Could you check a few things on this drawing? It's one solid part, dimensions in mm from its lowest x, y, z. A direction names the side the tool comes from. Round coordinates to 2 decimals unless told otherwise and drop trailing zeros. Loops run counter-clockwise (first coordinate to the right, second up) from the corner with the lowest first, then second, coordinate; pieces in that order, holes last. Notation, with made-up numbers: M 77,31 L 125,31 A23 cw 125,50 Z; hole C -38,82.5 d8. An arc over 180 degrees is marked long. Answer as CSV lines item,"result".
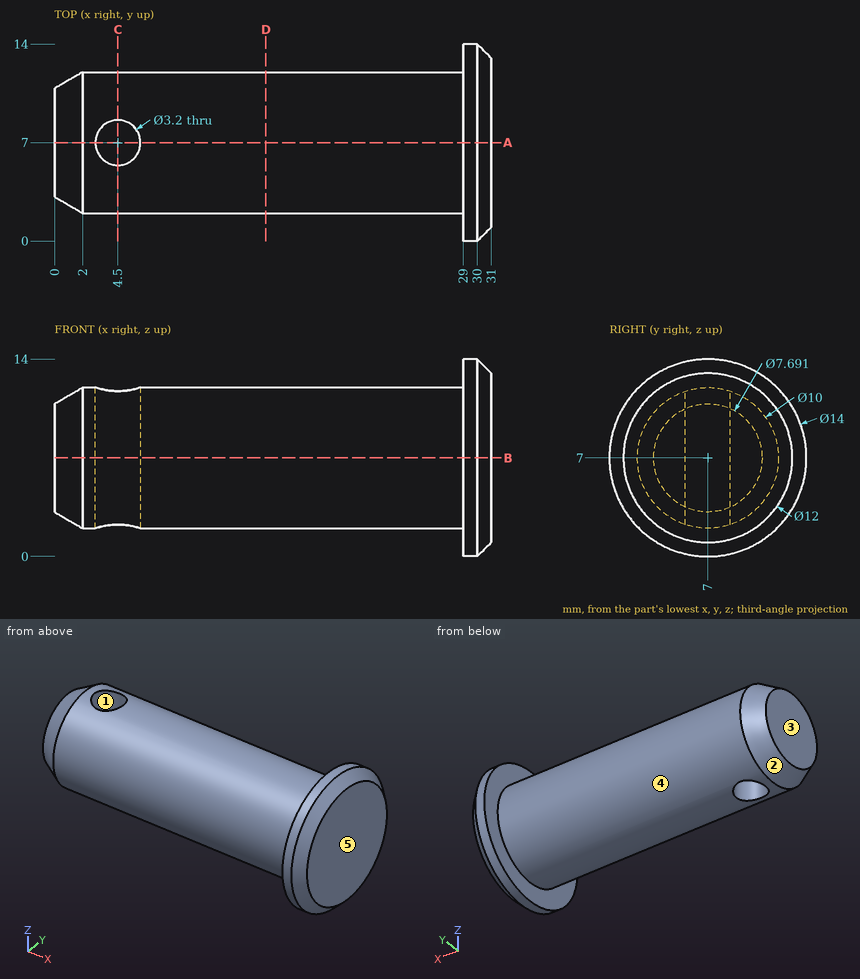
Item 1: If we section it at B-B on z = 7: Write out the boundary of the cut face in (x, y) (1 decimal), then the cut area to 3 significant figures.
Output:
outline,"M 0,3.2 L 2,2 L 29,2 L 29,0 L 30,0 L 31,1 L 31,13 L 30,14 L 29,14 L 29,12 L 2,12 L 0,10.8 Z; hole C 4.5,7 d3.2"
area,"307 mm2"
Item 2: If we section it at A-A on y = 7: Write out the boundary of the cut face in (x, z) (1 decimal).
Output:
outline,"M 0,3.2 L 2,2 L 2.9,2 L 2.9,12 L 2,12 L 0,10.8 Z; M 6.1,2 L 29,2 L 29,0 L 30,0 L 31,1 L 31,13 L 30,14 L 29,14 L 29,12 L 6.1,12 Z"
Item 3: If I drill on line 1 along X through (y, z) = (7, 7.5); line 2 along X through (y, z) = (7.75, 11.75) (1 decimal); line 3 along Y through (x, z) = (4.5, 9.5), over which ranges is the centre line in solid material (lowest first)? Write a range as from..to.
Output:
line 1,"x = 0..2.9, 6.1..31"
line 2,"x = 1.7..3.1, 5.9..31"
line 3,"y = 2.67..5.4, 8.6..11.33"
Item 4: If we section it at D-D on x = 15: Write out the boundary of the cut face in (y, z).
Output:
outline,"C 7,7 d10"
Item 5: If we section it at C-C on x = 4.5: Write out the boundary of the cut face in (y, z), then the cut area to 3 significant figures.
Output:
outline,"M 5.4,2.26 L 5.4,11.74 A5 ccw Z; M 8.6,2.26 A5 ccw 8.6,11.74 Z"
area,"47.1 mm2"
Item 6: Will these pins go through, and if not, where does the flat tip stop? pin 1 (4 mm diameter, centred on x = 26, y = 3, fed in from +Z); pin 2 (2 mm diameter, centred on x = 16.5, y = 3.5, fed in from +Z); pin 3 (7 mm diameter, centred on y = 4.5, z = 9.5, fed in from -X); pin 4 (4 mm diameter, centred on x = 10.5, z = 4, fed in from +Y).
Output:
pin 1,"stops at z = 11.58"
pin 2,"stops at z = 11.33"
pin 3,"stops at x = 0"
pin 4,"stops at y = 11.9"
Item 7: We'd pull the mould along Y, two halves only. Please class the marked faces 1, 2 and 3: released by +Y, released by -Y, zero draft, split by the parting line, or undercut.
Output:
face 1,"undercut"
face 2,"split by the parting line"
face 3,"zero draft"
Item 8: On a 3-axis mill with a long thin cutter (end or side, diameter ignored), from which of +Z, -Z, +X, -X, +Y, -Y can I reach the whole of each face in a straight line? I mean the marked faces 4 and 5. Say none if no direction works.
Output:
face 4,"-X"
face 5,"+Z, -Z, +X, +Y, -Y"
